Geometry: final body of the model. Coordinates: model frame, mm. A direction names the side the tool comes from. Coordinates: 2 decimals unless noted, no trailing zeros. Write each loop counter-clockwise with the first axis right and the second up, starting at its lowest first coordinate (ties: lowest second). Pieces come first, ordered by that corner, then holes. Notation, with made-up numbers: (42.25, 5) -> (72.25, 5) arc R12 ccw to (72.25, 9) -> close; hole circle Ø7 at (64.25, -39.5). An arc over 180 degrees is marked (long way). Answer as a JSON object with one key per item and string values. Group by question number.
```python
from build123d import *

# Parameters (mm, degrees)
F1_DEPTH  = 38
F3_DEPTH  = 25
F4_DEPTH  = 38
F0_W      = 25
F0_H      = 10
F5_DEPTH  = 5
F6_DEPTH  = 10
F0_W_2    = 8.5
F0_H_2    = 23
F7_DEPTH  = 25
F8_DEPTH  = 30
F9_DEPTH  = 20
F10_DEPTH = 15
F11_DEPTH = 35
F0_W_3    = 5
F0_H_3    = 28
F12_DEPTH = 38
F13_DEPTH = 14


with BuildPart() as f1:
    # F0 (on Top) → F1 (new body)
    with BuildSketch(Plane.XY):
        Polygon((-33.5, 19), (-38.5, 19), (-38.5, -24), (-33.5, -24), (-33.5, -14), (-33.5, -4), align=None)
    extrude(amount=F1_DEPTH)

    # F2 (on face) → F3 (cut)
    with BuildSketch(Plane.YZ.offset(-33.5)):
        Polygon((-24, 38), (-24, 14), (19, 38), align=None)
    extrude(amount=-F3_DEPTH, mode=Mode.SUBTRACT)

    # F0 (on Top) → F4 (join)
    with BuildSketch(Plane.XY):
        Polygon((8.5, 19), (8.5, 24), (-38.5, 24), (-38.5, 19), (-33.5, 19), (-8.5, 19), (0, 19), align=None)
    extrude(amount=F4_DEPTH)

    # F0 (on Top) → F5 (join)
    with BuildSketch(Plane.XY):
        with Locations((-21, -19)):
            Rectangle(F0_W, F0_H)
    extrude(amount=F5_DEPTH)

    # F0 (on Top) → F6 (join)
    with BuildSketch(Plane.XY):
        Polygon((33.5, -14), (33.5, -4), (8.5, -4), (0, -4), (-8.5, -4), (-33.5, -4), (-33.5, -14), (-8.5, -14), align=None)
    extrude(amount=F6_DEPTH)

    # F0 (on Top) → F7 (join)
    with BuildSketch(Plane.XY):
        with Locations((-4.25, 7.5)):
            Rectangle(F0_W_2, F0_H_2)
    extrude(amount=F7_DEPTH)

    # F0 (on Top) → F8 (join)
    with BuildSketch(Plane.XY):
        with Locations((4.25, 7.5)):
            Rectangle(F0_W_2, F0_H_2)
    extrude(amount=F8_DEPTH)

    # F0 (on Top) → F9 (join)
    with BuildSketch(Plane.XY):
        Polygon((-8.5, 19), (-33.5, 19), (-8.5, -4), align=None)
    extrude(amount=F9_DEPTH)

    # F0 (on Top) → F10 (join)
    with BuildSketch(Plane.XY):
        Polygon((-8.5, -4), (-33.5, 19), (-33.5, -4), align=None)
    extrude(amount=F10_DEPTH)

    # F0 (on Top) → F11 (join)
    with BuildSketch(Plane.XY):
        Polygon((33.5, -4), (33.5, 24), (8.5, 24), (8.5, 19), (8.5, -4), align=None)
    extrude(amount=F11_DEPTH)

    # F0 (on Top) → F12 (join)
    with BuildSketch(Plane.XY):
        with Locations((36, 10)):
            Rectangle(F0_W_3, F0_H_3)
    extrude(amount=F12_DEPTH)

    # F0 (on Top) → F13 (join)
    with BuildSketch(Plane.XY):
        Polygon((38.5, -24), (38.5, -4), (33.5, -4), (33.5, -14), (33.5, -24), align=None)
    extrude(amount=F13_DEPTH)


solid = f1.part
```
Item 1: Section C-C on z = 11. Output: boundary loops of the cut face in (x, y).
Item 2: Section D-D on y = 15.5. Output: boundary loops of the cut face in (x, z).
Item 3: Mould query, pull axis X, two halves, no side actions, for faces 6 (the flat face through (38.5, 5, 15)), 7 (the flat face through (33.5, 10, 36)), 8 (the flat face through (-1, 0, 0)). Classes: +X half, -X half, draft (parallel to the pull), parting line (faces both ways), or undercut.
Item 4: Set-up query: faces 1 (the flat face through (8.5, 21, 36)), 2 (the flat face through (-15, 22, 38)), 3 (the flat face through (36, -24, 7)), 4 (the flat face through (-35.965, -2.801, 25.832)), 5 (the flat face through (-33.5, -3, 21)). Return all of +Z, -Z, +X, -X, +Y, -Y with unobstructed straight access to the full face (end or side cutting, diameter ignored); none if empty.
Item 5: Section B-B on y = -20.5. Output: boundary loops of the cut face in (x, z).
Item 6: Contact query for flat-ended pins moving along their axis: pin 1 (2.5 mm diameter, centred on x = 4, y = 12.5, fed in from +Z); pin 2 (11.5 mm diameter, centred on x = -21, y = 3.5, fed in from +Z); pin 3 (22.5 mm diameter, centred on x = 9, z = 25, fed in from -Y); pin 4 (4 mm diameter, centred on x = -23, y = -15.5, fed in from -Z). Output: stop coordinate, or through.
Item 7: Ray query, L1, parallel to X at y = 5.5, z = 28; L2, parallel to Z at x = 12.5, y = -7; L3, parallel to Y at x = -18, z = 6. Return the intervals inside material, ascending. Write a range as [from, to].
Item 8: Section A-A on x = -27. Output: boundary loops of the cut face in (y, z).
Answer sheet:
{
 "1": {"outline": "(-38.5, -24) -> (-33.5, -24) -> (-33.5, -4) -> (33.5, -4) -> (33.5, -24) -> (38.5, -24) -> (38.5, 24) -> (-38.5, 24) -> close"},
 "2": {"outline": "(-38.5, 0) -> (38.5, 0) -> (38.5, 38) -> (33.5, 38) -> (33.5, 35) -> (8.5, 35) -> (8.5, 30) -> (0, 30) -> (0, 25) -> (-8.5, 25) -> (-8.5, 20) -> (-29.7, 20) -> (-29.7, 15) -> (-33.5, 15) -> (-33.5, 36.05) -> (-38.5, 36.05) -> close"},
 "3": {"face 6": "+X half", "face 7": "undercut", "face 8": "draft"},
 "4": {"face 1": "+Z, +Y, -Y", "face 2": "+Z, +X, -X, +Y, -Y", "face 3": "+Z, -Z, +X, -X, -Y", "face 4": "+Z, -X, -Y", "face 5": "+Z, -Y"},
 "5": {"outline": "(-38.5, 0) -> (-8.5, 0) -> (-8.5, 5) -> (-33.5, 5) -> (-33.5, 15.95) -> (-38.5, 15.95) -> close; (33.5, 0) -> (38.5, 0) -> (38.5, 14) -> (33.5, 14) -> close"},
 "6": {"pin 1": "stops at z = 30", "pin 2": "stops at z = 20", "pin 3": "stops at y = -4", "pin 4": "stops at z = 0"},
 "7": {"L1": "x = [-38.5, -33.5], [0, 38.5]", "L2": "z = [0, 10]", "L3": "y = [-14, 24]"},
 "8": {"outline": "(-24, 0) -> (24, 0) -> (24, 38) -> (19, 38) -> (19, 20) -> (13.02, 20) -> (13.02, 15) -> (-4, 15) -> (-4, 10) -> (-14, 10) -> (-14, 5) -> (-24, 5) -> close"}
}
